```python
from build123d import *

# Parameters (mm, degrees)
F1_R     = 30
F1_R_2   = 25
F3_R     = 82.5
F3_R_2   = 9
F3_R_3   = 25
F4_DEPTH = 15
F5_R     = 82.5
F5_R_2   = 9
F5_R_3   = 25
F6_DEPTH = 15


with BuildPart() as f2:
    # F2: sweep along a path in F0
    with BuildLine(Plane.YZ) as f2_path:
        Line((0, 0), (0, -395))
        ThreePointArc((0, -395), (-29.289322, -465.710678), (-100, -495))
        Line((-100, -495), (-930, -495))
    # F1 (on Top) → F2 (sweep)
    with BuildSketch(Plane.XY):
        Circle(F1_R)
        Circle(F1_R_2, mode=Mode.SUBTRACT)
    sweep(path=f2_path.line)

    # F3 (on Top) → F4 (join)
    with BuildSketch(Plane.XY):
        Circle(F3_R)
        with Locations((0, -62.5)):
            Circle(F3_R_2, mode=Mode.SUBTRACT)
        with Locations((-62.5, 0)):
            Circle(F3_R_2, mode=Mode.SUBTRACT)
        Circle(F3_R_3, mode=Mode.SUBTRACT)
        with Locations((62.5, 0)):
            Circle(F3_R_2, mode=Mode.SUBTRACT)
        with Locations((0, 62.5)):
            Circle(F3_R_2, mode=Mode.SUBTRACT)
    extrude(amount=-F4_DEPTH)

    # F5 (on face) → F6 (join)
    with BuildSketch(Plane.XZ.offset(930)):
        with Locations((0, -495)):
            Circle(F5_R)
        with Locations((-62.5, -495)):
            Circle(F5_R_2, mode=Mode.SUBTRACT)
        with Locations((0, -557.5)):
            Circle(F5_R_2, mode=Mode.SUBTRACT)
        with Locations((0, -495)):
            Circle(F5_R_3, mode=Mode.SUBTRACT)
        with Locations((0, -432.5)):
            Circle(F5_R_2, mode=Mode.SUBTRACT)
        with Locations((62.5, -495)):
            Circle(F5_R_2, mode=Mode.SUBTRACT)
    extrude(amount=-F6_DEPTH)


solid = f2.part
```
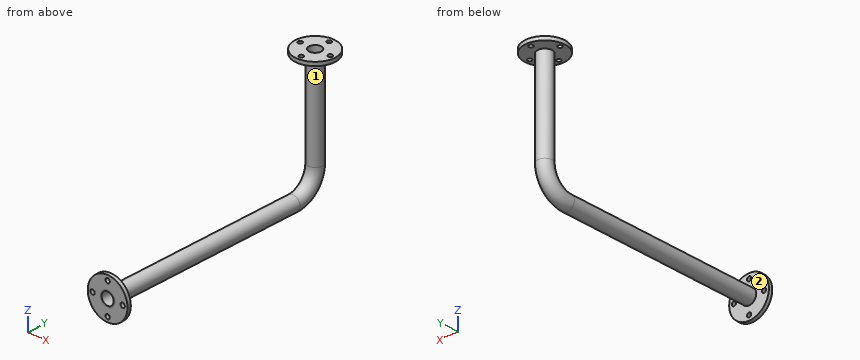
Can you work these out from the model? Positions are in its coordinate system, mm. Face numbers are marked on the shaded views. Give positions to 0.01 mm unless a question says otherwise; leave off trailing zeros. Loops run counter-clockwise (first coordinate to the right, second up) from the corner with the lowest first, then second, coordinate; pieces in that order, holes last. Notation, with made-up numbers: M 17.5,-1.5 L 53.5,-1.5 A27 cw 53.5,26.5 Z; hole C 71,25 d8. An arc over 180 degrees is marked long. Use one line per item in the form item = value. Start each with the question number.
(1) Please list where these lines run through material, in increasing order: line 1 (Z direction, x = 0, y = -921.5); line 2 (Y direction, x = 0, z = -11.5); line 3 (Y direction, x = -18, z = -459.5).
(2) I'm going to push flat-ended pins straight in: P1, Ø14.5, axis at x = 0, z = -432.5, coming from the -Y side; P2, Ø23.5, axis at x = 0, y = -62.5, coming from the -Z side; P3, Ø6, axis at y = -590.5, z = -469, coming from the -X side. Where does each tip first touch, or does it pass through?
(3) Thinking about a two-plate mould opening in Z: for the marked faces 1 and 2, which applies, released by +Z, released by -Z, zero draft, split by the parting line, or undercut?
(4) I want a section at A-A, the plane z = -57. Write out the boundary of the cut face in (x, y), and give its area (3 significant figures).
Worked out:
q1.line_1 = -577.5 to -566.5, -548.5 to -520, -470 to -441.5, -423.5 to -412.5
q1.line_2 = -82.5 to -71.5, -53.5 to -25, 25 to 53.5, 71.5 to 82.5
q1.line_3 = -930 to -915, -59.8 to -48.32, -1.97 to 5.9
q2.P1 = -46.17
q2.P2 = -522.42
q2.P3 = -19.26
q3.face_1 = undercut
q3.face_2 = zero draft
q4.outline = C 0,0 d60; hole C 0,0 d50
q4.area = 864 mm²
